Could you check a few things on this model? Use its own coordinates, in mm. A direction names the side the tool comes from. Coordinates: 2 decimals unless noted, no trailing zeros. Write each loop counter-clockwise with the first axis right and the second up, starting at its lowest first coordinate (ties: lowest second). Pieces come first, ordered by that corner, then holes.
Item 1: Which directions (+Z, -Z, +X, -X, +Y, -Y) give clear straight access to the entire face, cutting with the end or side of a thin tool? Please do faces 4 (the flat face through (5, 3, -2)), 5 (the flat face through (1, 2, 2)).
Item 2: If I drill on probe 1 along X at (y, z) = (2.55, 0); probe 2 along X at (y, z) = (1.9, 0); probe 3 along Y at (x, z) = (-3.25, 0.25), over which ranges is the centre line in solid material (lowest first)?
Item 3: Thinking about a two-plate mould opening in Z: for faces 1 (the cylindrical face through (-6.324, 1.521, -4.032)), 2 (the cylindrical face through (2, 1, 0)), 3 (the flat face through (2, 0, 2)), which applies, +Z half, -Z half, draft (parallel to the pull), parting line (faces both ways), or undercut?
Item 4: I want a section at D-D on z = 6. Please give me the cut outline in (x, y), then the cut area to 3 significant figures.
Item 5: I want a section at C-C on y = 1.3. Please give me the cut outline in (x, z).
Item 6: For P1, Ø6.5, axis at x = 0, z = 0, coming from the +Y side, with a flat end and sliding along its axis, tell me the tip position at first contact or that it passes through.
from build123d import *

# Parameters (mm, degrees)
FILLET_1_R = 0.5


with BuildPart() as part:
    # 草图2 → 旋转1 (revolve)
    with BuildSketch(Plane.XY, mode=Mode.PRIVATE) as revolve_1_sk:
        Polygon((2, 0), (7.5, 0), (7.5, 3), (4.5, 3), (4.5, 2), (2, 2), align=None)
    revolve(revolve_1_sk.sketch.rotate(Axis((0, 0, 0), (0, 1, 0)), 90), axis=Axis((0, 0, 0), (0, 1, 0)))

    # 圆角1
    fillet_1_edges = [part.edges().sort_by_distance(p)[0] for p in [
        (0, 2, 4.5),
        (0, 3, 4.5),
    ]]
    fillet(fillet_1_edges, radius=FILLET_1_R - 0.0001)  # a hair under: the kernel refuses the full size


solid = part.part
Response values:
1. face 4: +Z, -Z, +X, -X, +Y
1. face 5: +Y
2. probe 1: x = -7.5 to -4.5, 4.5 to 7.5
2. probe 2: x = -7.5 to -2, 2 to 7.5
2. probe 3: y = 0 to 2
3. face 1: parting line
3. face 2: undercut
3. face 3: draft
4. outline: (-4.5, 0) - (4.5, 0) - (4.5, 3) - (-4.5, 3) - close
4. area: 27.0 mm2
5. outline: circle Ø15 at (0, 0); hole circle Ø4 at (0, 0)
6. P1: stops at y = 2
